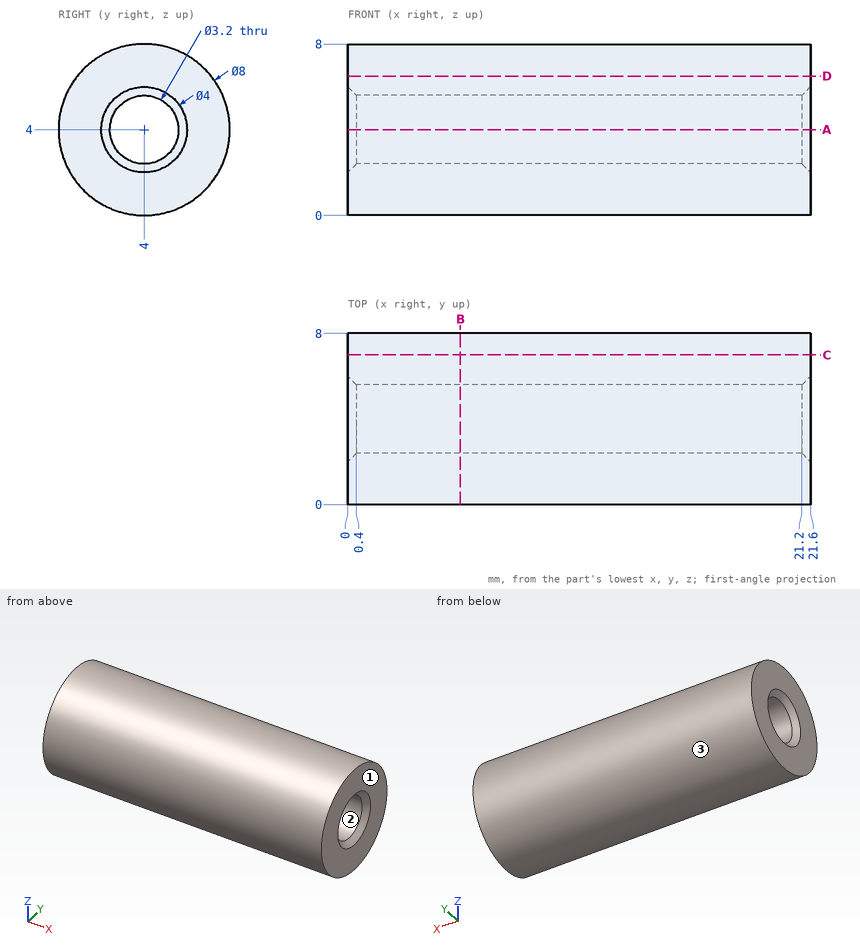
The figure shows three views and two pictorial views of one solid part (mm, origin at its lowest corner). Answer the questions. Round coordinates to 2 decimals unless told otherwise and drop trailing zeros. Write each loop counter-clockwise with the first axis right and the second up, starting at its lowest first coordinate (ties: lowest second). Pieces come first, ordered by that corner, then holes. Notation, with made-up numbers: M -11.5,68 L 44.5,68 A19 ccw 44.5,87 Z; hole C 69.5,-20 d7. An arc over 180 degrees is marked long. Use a Markdown table: item, result.
1) The part is cut by section B-B on x = 5.25. Give the vertices of the cut face in (y, z), plus the area to 3 significant figures.
Taken from the geometry:
| item | result |
|---|---|
| outline | C 4,4 d8; hole C 4,4 d3.2 |
| area | 42.2 mm2 |
2) Consider line 1 (Y direction, x = 9.5, z = 4); line 2 (Z direction, x = 8.5, y = 3); line 3 (Z direction, x = 12.75, y = 3.25). Determine where each line is inside the solid, lowest interval first. Write a range as [from, to].
Taken from the geometry:
| item | result |
|---|---|
| line 1 | y = [0, 2.4], [5.6, 8] |
| line 2 | z = [0.13, 2.75], [5.25, 7.87] |
| line 3 | z = [0.07, 2.59], [5.41, 7.93] |
3) The part is cut by section D-D on z = 6.5. Give the vertices of the cut face in (x, y).
Taken from the geometry:
| item | result |
|---|---|
| outline | M 0,0.88 L 21.6,0.88 L 21.6,7.12 L 0,7.12 Z |
4) The part is cut by section A-A on z = 4. Give the vertices of the cut face in (x, y).
Taken from the geometry:
| item | result |
|---|---|
| outline | M 0,0 L 21.6,0 L 21.6,2 L 21.2,2.4 L 0.4,2.4 L 0,2 Z; M 0,6 L 0.4,5.6 L 21.2,5.6 L 21.6,6 L 21.6,8 L 0,8 Z |
5) Determine the mould class of the marked faces 1, 2 and 3 for opening direction Z: pulls with the +Z half, pulls with the -Z half, needs draft (parallel to the pull), parting line crosses it, or undercut.
Taken from the geometry:
| item | result |
|---|---|
| face 1 | needs draft |
| face 2 | undercut |
| face 3 | parting line crosses it |
6) The part is cut by section C-C on y = 7. Give the vertices of the cut face in (x, z).
Taken from the geometry:
| item | result |
|---|---|
| outline | M 0,1.35 L 21.6,1.35 L 21.6,6.65 L 0,6.65 Z |
